from build123d import *

# Parameters (mm, degrees)
F1_W     = 152.4
F1_H     = 152.4
F2_DEPTH = 76.2
F4_DEPTH = 25.4
F6_DEPTH = 25.4


# Not quite as in the source:
# - a variable given as a bare number and used for a length is read in inches; the dataset says mm whatever the document's units were


with BuildPart() as f2:
    # F1 (on Front) → F2 (new body, symmetric)
    with BuildSketch(Plane.XZ):
        Rectangle(F1_W, F1_H)
    extrude(amount=F2_DEPTH, both=True)

    # F3 (on face) → F4 (cut)
    with BuildSketch(Plane.XZ.offset(76.2)):
        Polygon((19.1713254899, 46.1731813848), (-48.0633080006, 46.1731813848), (-48.0633080006, -39.9627536535), (-36.4525094628, -39.1526967287), (-36.4525094628, 0), (-9.720666334, 0), (-9.720666334, 9.9906884134), (-36.7225259542, 9.9906884134), (-36.7225259542, 34.5623828471), (19.1713254899, 34.5623828471), align=None)
    extrude(amount=-F4_DEPTH, mode=Mode.SUBTRACT)

    # F5 (on face) → F6 (join)
    with BuildSketch(Plane(origin=(0, 76.2, 0), x_dir=(-1, 0, 0), z_dir=(0, 1, 0))):
        Polygon((48.0633080006, -39.9627536535), (48.0633080006, 46.1731813848), (-19.1713254899, 46.1731813848), (-19.1713254899, 34.5623828471), (36.7225259542, 34.5623828471), (36.7225259542, 9.9906884134), (9.720666334, 9.9906884134), (9.720666334, 0), (36.4525094628, 0), (36.4525094628, -39.1526967287), align=None)
    extrude(amount=F6_DEPTH)


solid = f2.part
Design review of the part built by this model. Coordinates are the model's own, in mm. A direction names the side the tool comes from. Give positions to 0.01 mm unless a question says otherwise; leave off trailing zeros. Loops run counter-clockwise (first coordinate to the right, second up) from the corner with the lowest first, then second, coordinate; pieces in that order, holes last. Notation, with made-up numbers: M 44,-28.5 L 73,-28.5 A20 ccw 73,-5.5 Z; hole C 9.5,-23.5 d6. An arc over 180 degrees is marked long. Write item = value, one per line.
Q1. Insertion check: pin 1 (8 mm diameter, centred on x = 47, y = 82.5, fed in from -Z); pin 2 (12.5 mm diameter, centred on x = -12.5, y = 87, fed in from -Z); pin 3 (8 mm diameter, centred on y = 84, z = 3, fed in from +X); pin 4 (7.5 mm diameter, centred on y = 85.5, z = -16, fed in from +X). Each pin has a flat end and moves straight along its axis. Give the tip position at first contact, or say it passes through.
Output values:
pin_1 = through
pin_2 = 0
pin_3 = -9.72
pin_4 = -36.45
Q2. We need section A-A (x = -32). Give the boundary of the cut face in (y, z).
Output values:
outline = M -76.2,-76.2 L 76.2,-76.2 L 76.2,0 L 101.6,0 L 101.6,9.99 L 76.2,9.99 L 76.2,34.56 L 101.6,34.56 L 101.6,46.17 L 76.2,46.17 L 76.2,76.2 L -76.2,76.2 L -76.2,46.17 L -50.8,46.17 L -50.8,34.56 L -76.2,34.56 L -76.2,9.99 L -50.8,9.99 L -50.8,0 L -76.2,0 Z
Q3. We need section B-B (z = -59.5). Give the boundary of the cut face in (x, y), plus the area to 3 significant figures.
Output values:
outline = M -76.2,-76.2 L 76.2,-76.2 L 76.2,76.2 L -76.2,76.2 Z
area = 23,200 mm^2
Q4. For faces 1 (the flat face through (-8, 89, 34.562)), 2 (the flat face through (-15, 89, 46.173)), 3 (the flat face through (-42.177, 88.722, -39.552)), 4 (the flat face through (-36.723, -64, 22)), list the 3-axis set-ups (+Z, -Z, +X, -X, +Y, -Y) from which the entire face can be reached by the end or side of a thin tool; tool diameter is ignored.
Output values:
face_1 = +X, +Y
face_2 = +Z, +X, -X, +Y
face_3 = -Z, +X, +Y
face_4 = -Y
Q5. To check wall thickness, follow line 1 (X direction, y = -60, z = 43.5); line 2 (Y direction, x = 23, z = 16); line 3 (Z direction, x = -47, y = 84.5). State the ranges of each line that lie inside material, in increasing order. Write a range as [from, to].
Output values:
line_1 = [-76.2, -48.06], [19.17, 76.2]
line_2 = [-76.2, 76.2]
line_3 = [-39.89, 46.17]
Q6. Draft analysis for pull direction X (two halves, no side actions). For faces 5 (the flat face through (-36.453, 89, -19)), 6 (the flat face through (-24.2, 101.6, 9.7)), 7 (the flat face through (-42.339, -63.678, -39.563)), state which applies: +X half, -X half, draft (parallel to the pull), parting line (faces both ways), or undercut.
Output values:
face_5 = +X half
face_6 = draft
face_7 = undercut
